Source: CAD feature listing. Evaluate the final solid. Frame: model axes, mm. Give positions to 0.01 mm unless a question says otherwise; leave off trailing zeros. Use one line per item in the form item = value. Start each with the question number.
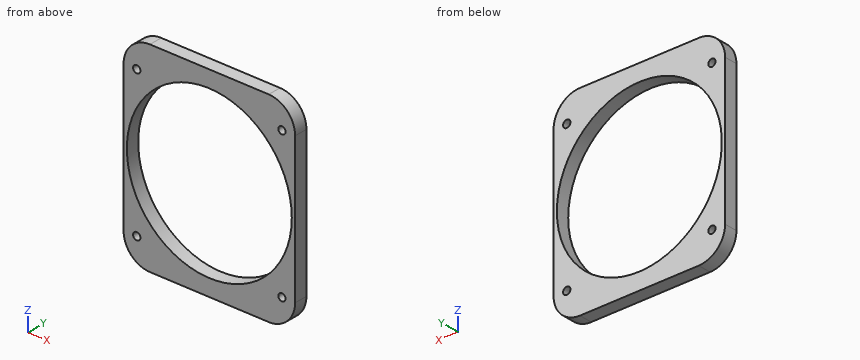
from build123d import *

# Parameters (mm, degrees)
SKETCH1_W           = 82.55
SKETCH1_H           = 95.25
SKETCH1_R           = 38.1
SKETCH1_R_2         = 1.75
BOSS_EXTRUDE1_DEPTH = 6.35
FILLET1_R           = 12.7
SKETCH2_R           = 39.6875
SKETCH2_R_2         = 38.1
CUT_EXTRUDE1_DEPTH  = 7.35


with BuildPart() as part:
    # Sketch1 → Boss-Extrude1 (new body)
    with BuildSketch(Plane(origin=(0, 0, 0), x_dir=(1, 0, 0), z_dir=(0, 1, 0))):
        Rectangle(SKETCH1_W, SKETCH1_H)
        Circle(SKETCH1_R, mode=Mode.SUBTRACT)
        with Locations((-34.925, 34.925)):
            Circle(SKETCH1_R_2, mode=Mode.SUBTRACT)
        with Locations((-34.925, -34.925)):
            Circle(SKETCH1_R_2, mode=Mode.SUBTRACT)
        with Locations((34.925, -34.925)):
            Circle(SKETCH1_R_2, mode=Mode.SUBTRACT)
        with Locations((34.925, 34.925)):
            Circle(SKETCH1_R_2, mode=Mode.SUBTRACT)
    extrude(amount=BOSS_EXTRUDE1_DEPTH)

    # Fillet1
    fillet1_edges = [part.edges().sort_by_distance(p)[0] for p in [
        (-41.275, 3.175, -47.625),
        (41.275, 3.175, -47.625),
        (41.275, 3.175, 47.625),
        (-41.275, 3.175, 47.625),
    ]]
    fillet(fillet1_edges, radius=FILLET1_R)

    # Sketch2 → Cut-Extrude1 (cut, through all)
    with BuildSketch(Plane(origin=(0, 6.35, 0), x_dir=(1, 0, 0), z_dir=(0, 1, 0))):
        Circle(SKETCH2_R)
        Circle(SKETCH2_R_2, mode=Mode.SUBTRACT)
    extrude(amount=-CUT_EXTRUDE1_DEPTH, mode=Mode.SUBTRACT)


solid = part.part
1) Pin query (flat end, axial travel): pin 1 (5.5 mm diameter, centred on x = 34.925, z = 34.925, fed in from +Y). Return the tip coordinate at first contact, or that it passes through.
2) Material intervals for probe 1 along X at (y, z) = (2.5, -1) (3 decimals); probe 2 along X at (y, z) = (1.25, 5) (3 decimals); probe 3 along Z at (x, y) = (14.5, 5) (3 decimals), sorted ascending.
3) Cut plane A-A, the plane y = 3.75. Count the separate pieces of the cut face and the enclosed holes in it, plus the area to 3 significant figures.
Output values:
q1.pin_1 = 6.35
q2.probe_1 = -41.275 to -39.675, 39.675 to 41.275
q2.probe_2 = -41.275 to -39.371, 39.371 to 41.275
q2.probe_3 = -47.625 to -36.944, 36.944 to 47.625
q3.separate_pieces = 1
q3.enclosed_holes = 5
q3.area = 2,740 mm^2
